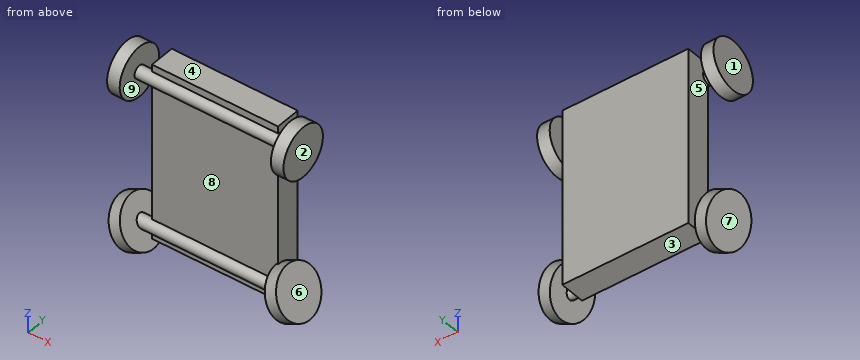
from build123d import *

# Parameters (mm, degrees)
CROQUIS2_W                 = 50
CROQUIS2_H                 = 70
SALIENTE_EXTRUIR1_DEPTH    = 10
CROQUIS4_R                 = 2.5
SALIENTE_EXTRUIR2_DEPTH    = 30
CROQUIS5_R                 = 10
SALIENTE_EXTRUIR3_DEPTH    = 5
CORTAR_EXTRUIR1_DEPTH      = 5
CORTAR_EXTRUIR1_DEPTH_BACK = 5
CROQUIS8_R                 = 10
SALIENTE_EXTRUIR4_DEPTH    = 5
CROQUIS9_R                 = 10
SALIENTE_EXTRUIR5_DEPTH    = 5


with BuildPart() as part:
    # Croquis2 → Saliente-Extruir1 (new body)
    with BuildSketch(Plane(origin=(0, 0, 0), x_dir=(1, 0, 0), z_dir=(0, 1, 0))):
        Rectangle(CROQUIS2_W, CROQUIS2_H)
    extrude(amount=SALIENTE_EXTRUIR1_DEPTH)

    # Croquis4 → Saliente-Extruir2 (add, symmetric)
    with BuildSketch(Plane(origin=(0, 0, 0), x_dir=(0, 0, -1), z_dir=(1, 0, 0))):
        with Locations((-29.646809276, 0)):
            Circle(CROQUIS4_R)
    saliente_extruir2 = extrude(amount=SALIENTE_EXTRUIR2_DEPTH, both=True)

    # Croquis5 → Saliente-Extruir3 (add)
    with BuildSketch(Plane(origin=(30, 0, 0), x_dir=(0, 0, -1), z_dir=(1, 0, 0))):
        with Locations((-29.646809276, 0)):
            Circle(CROQUIS5_R)
    saliente_extruir3 = extrude(amount=SALIENTE_EXTRUIR3_DEPTH)

    # Simetría1: Saliente-Extruir3 across plane
    add(saliente_extruir3.mirror(Plane(origin=(0, 0, 0), x_dir=(0, 0, 1), z_dir=(1, 0, 0))))

    # Simetría2: Saliente-Extruir2 across plane
    add(saliente_extruir2.mirror(Plane.XY))

    # Croquis7 → Cortar-Extruir1 (cut, two sides: drawn at the far end of the back side and taken through both)
    with BuildSketch(Plane(origin=(0, 0, 0), x_dir=(1, 0, 0), z_dir=(0, 1, 0)).offset(-CORTAR_EXTRUIR1_DEPTH_BACK)):
        Polygon((-30, 27.146809276), (-27.5, 32.146809276), (-30, 32.146809276), align=None)
        Polygon((30, 32.146809276), (27.5, 27.146809276), (30, 27.146809276), align=None)
    extrude(amount=CORTAR_EXTRUIR1_DEPTH + CORTAR_EXTRUIR1_DEPTH_BACK, mode=Mode.SUBTRACT)

    # Croquis8 → Saliente-Extruir4 (add)
    with BuildSketch(Plane(origin=(11.14127629, 0, 5.570638145), x_dir=(0.4472135954999586, 0, -0.8944271909999156), z_dir=(0.8944271909999156, 0, 0.4472135954999586))):
        with Locations(Location((39.374303213, 0, 0), (0, 0, 180))):
            Circle(CROQUIS8_R)
    extrude(amount=SALIENTE_EXTRUIR4_DEPTH)

    # Croquis9 → Saliente-Extruir5 (add)
    with BuildSketch(Plane(origin=(-34.85872371, 0, -17.429361855), x_dir=(-0.44721359549995665, 0, 0.8944271909999165), z_dir=(-0.8944271909999165, 0, -0.44721359549995665))):
        with Locations((-13.659521472, 0)):
            Circle(CROQUIS9_R)
    extrude(amount=SALIENTE_EXTRUIR5_DEPTH)


solid = part.part
CAD build for the part. Positions are in the model's coordinates, mm. Face numbers are marked on the shaded views. A direction names the side the tool comes from. Round coordinates to 2 decimals unless told otherwise and drop trailing zeros. Loops run counter-clockwise (first coordinate to the right, second up) from the corner with the lowest first, then second, coordinate; pieces in that order, holes last.
(1) Cut at A-A (x = 5.5). Give the cut face in (y, z), plus the area to 3 significant figures.
(2) Two-plate mould, pull along X, no slides. Class the marked faces 1, 2, 3 and 4: +X half, -X half, draft (parallel to the pull), parting line (faces both ways), or undercut.
(3) Cut at B-B (z = 24). Give the cut face in (x, y).
(4) Drop flat-ended pins along their axis: pin 1 (12 mm diameter, centred on y = -1, z = -4, fed in from +X); pin 2 (6 mm diameter, centred on y = -4.5, z = 25, fed in from -X); pin 3 (10 mm diameter, centred on x = 14, y = -3.5, fed in from +Z); pin 4 (12 mm diameter, centred on x = -27.5, y = 0.5, fed in from +Z). Give the stop position or say it passes through.
(5) Cut at C-C (y = -3.75). Give the cut face in (x, z).
(6) Which spindle directions (+Z, -Z, +X, -X, +Y, -Y) get a long thin tool onto all of the face, cutting with end or side? Do the marked faces 5, 6, 7, 8 and 9. Say none if no direction does.
(7) Cut at D-D (y = 7.25). Give the cut face in (x, z).
(8) Wall check: line 1 along X through (y, z) = (1.75, 24); line 2 along X through (y, z) = (1, -26); line 3 along Z through (x, y) = (27, 1.25). Give the ranges that are in metal, low to high.
Findings below:
1. outline: (0, -35) - (10, -35) - (10, 35) - (0, 35) - (0, 32.15) arc R2.5 ccw to (0, 27.15) - (0, -27.15) arc R2.5 ccw to (0, -32.15) - close
1. area: 720 mm2
2. face 1: -X half
2. face 2: +X half
2. face 3: undercut
2. face 4: undercut
3. outline: (-35, -8.25) - (-30, -8.25) - (-30, 8.25) - (-35, 8.25) - close; (-25, 0) - (25, 0) - (25, 10) - (-25, 10) - close; (30, -8.25) - (35, -8.25) - (35, 8.25) - (30, 8.25) - close
4. pin 1: stops at x = 25
4. pin 2: stops at x = -35
4. pin 3: stops at z = 35
4. pin 4: stops at z = 39.65
5. outline: (-37.37, -23.59) - (-29.08, -40.17) - (-24.6, -37.94) - (-32.9, -21.36) - close; (-35, 20.38) - (-30, 20.38) - (-30, 38.92) - (-35, 38.92) - close; (24.6, -21.36) - (32.9, -37.94) - (37.37, -35.7) - (29.08, -19.12) - close; (30, 20.38) - (35, 20.38) - (35, 38.92) - (30, 38.92) - close
6. face 5: +Y
6. face 6: +X, +Y, -Y
6. face 7: -Z, -X, +Y, -Y
6. face 8: -Y
6. face 9: none
7. outline: (-36.3, -25.72) - (-30.14, -38.04) - (-25.67, -35.81) - (-31.83, -23.49) - close; (-35, 22.76) - (-30, 22.76) - (-30, 36.53) - (-35, 36.53) - close; (-25, -35) - (25, -35) - (25, 35) - (-25, 35) - close; (25.67, -23.49) - (31.83, -35.81) - (36.3, -33.57) - (30.14, -21.25) - close; (30, 22.76) - (35, 22.76) - (35, 36.53) - (30, 36.53) - close
8. line 1: x = -35 to -30, -25 to 25, 30 to 35
8. line 2: x = -36.16 to -30.57, -25 to 25, 26.93 to 32.52
8. line 3: z = -31.81 to -27.48, -26.15 to -19.43, 27.48 to 31.81
